Geometry: see drawing. Coordinates: mm, zero at the bounding-box minimum. A direction names the side the tool comes from. Coordinates: 2 decimals unless noted, no trailing zeros. Write each loop counter-clockwise with the first axis right and the second up, starting at its lowest first coordinate (ties: lowest second). Pieces come first, ordered by that corner, then holes. Notation, with made-up numbers: (-9.5, -38.5) - (18.5, -38.5) arc R22 cw to (18.5, -2.5) - close; hole circle Ø1 at (-2.75, 7). An arc over 180 degrees is marked (long way). Use CSV: the item, a comma, the result in double quotes.
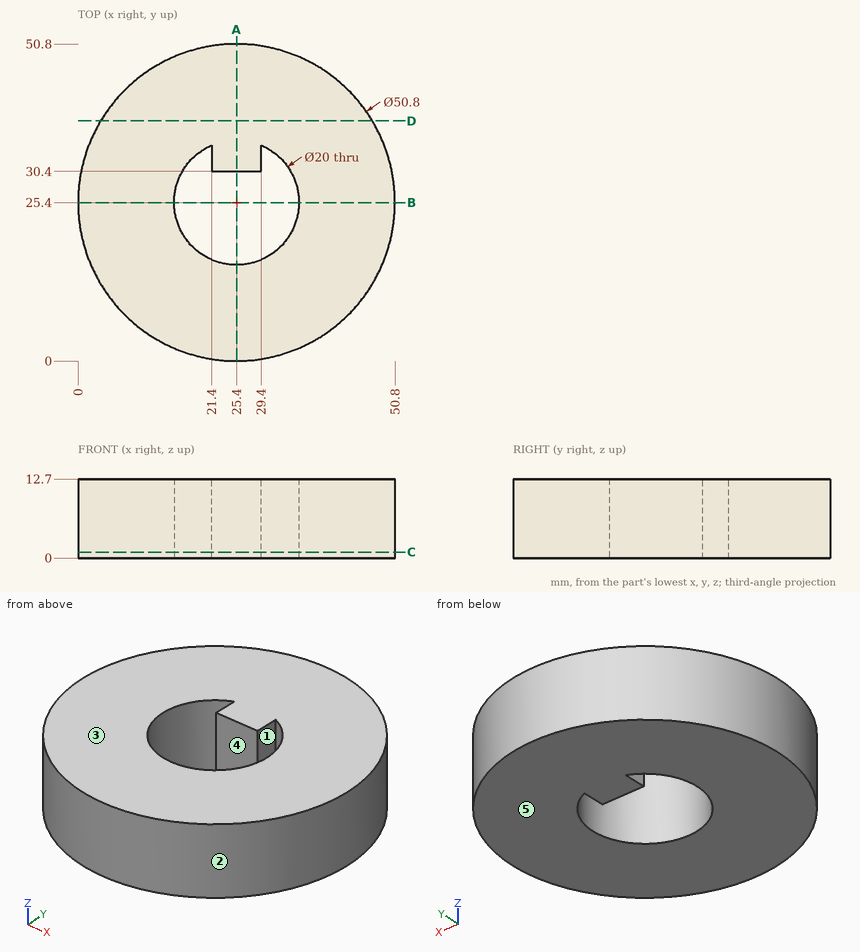
(1) Draft query along X for the marked faces 1, 2 and 3. Return one class per face: pulls with the +X half, pulls with the -X half, needs draft (parallel to the pull), parting line crosses it, or undercut.
Check values:
face 1,"undercut"
face 2,"parting line crosses it"
face 3,"needs draft"
(2) Ray query, probe 1 along Y at (x, z) = (25.4, 9.5); probe 2 along X at (y, z) = (32, 1.25); probe 3 along X at (y, z) = (25, 0.5). Return the intervals inside material, ascending. Write a range as from..to.
Check values:
probe 1,"0..15.4, 30.4..50.8"
probe 2,"0.87..17.89, 21.4..29.4, 32.91..49.93"
probe 3,"0..15.41, 35.39..50.8"
(3) Pin query (flat end, axial travel): pin 1 Ø1.5 at (y, z) = (13.5, 10.5) entering from -X; pin 2 Ø2 at (y, z) = (36, 5) entering from -X; pin 3 Ø1.2 at (y, z) = (32.5, 7) entering from -X. Return the tip coordinate at first contact, or that it passes through.
Check values:
pin 1,"x = 2.58"
pin 2,"x = 1.88"
pin 3,"x = 0.85"
(4) Cut plane B-B on y = 25.4. Return loops of the section in (x, z), and give its area (3 significant figures).
Check values:
outline,"(0, 0) - (15.4, 0) - (15.4, 12.7) - (0, 12.7) - close; (35.4, 0) - (50.8, 0) - (50.8, 12.7) - (35.4, 12.7) - close"
area,"391 mm^2"
(5) Cut plane D-D on y = 38.5. Return loops of the section in (x, z).
Check values:
outline,"(3.64, 0) - (47.16, 0) - (47.16, 12.7) - (3.64, 12.7) - close"
(6) Reachability of the marked faces 4 and 5 from +Z, -Z, +X, -X, +Y, -Y: full face, straight path, thin tool, end or side. Return the list, or none.
Check values:
face 4,"+Z, -Z"
face 5,"-Z, +X, -X, +Y, -Y"
(7) Cut plane C-C on z = 1. Return loops of the section in (x, y), and give its area (3 significant figures).
Check values:
outline,"circle Ø50.8 at (25.4, 25.4); hole (21.4, 30.4) - (21.4, 34.57) arc R10 ccw (long way) to (29.4, 34.57) - (29.4, 30.4) - close"
area,"1,750 mm^2"
(8) Cut plane A-A on x = 25.4. Return loops of the section in (y, z).
Check values:
outline,"(0, 0) - (15.4, 0) - (15.4, 12.7) - (0, 12.7) - close; (30.4, 0) - (50.8, 0) - (50.8, 12.7) - (30.4, 12.7) - close"
